Source: three-view drawing plus pictorial views. Frame: mm from the lowest corner of the part. Coordinates: 2 decimals unless noted, no trailing zeros. Write each loop counter-clockwise with the first axis right and the second up, starting at its lowest first coordinate (ties: lowest second). Pieces come first, ordered by that corner, then holes. Notation, with made-up numbers: (68.5, -20) - (99.5, -20) arc R19 ccw to (99.5, -1) - close; hole circle Ø3 at (-27, 53). An arc over 180 degrees is marked (long way). One line per item, written item: value.
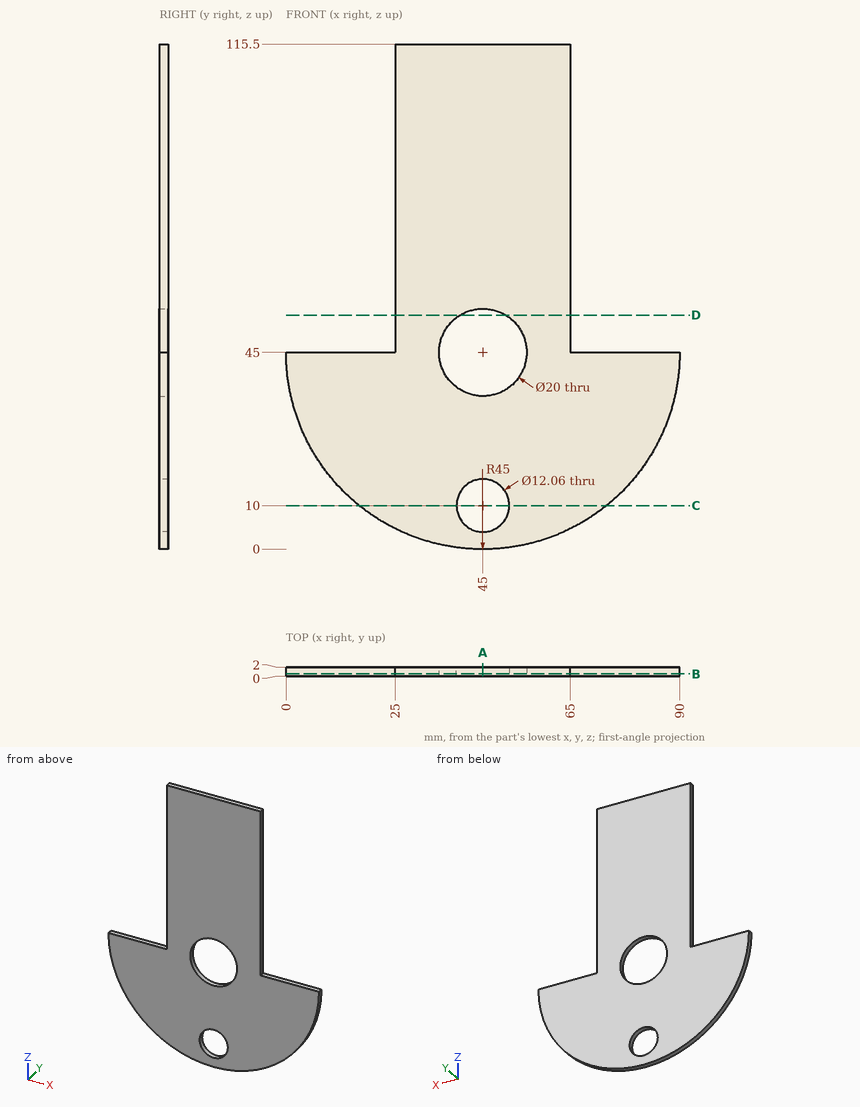
1) Material intervals for line 1 (Z direction, x = 45, y = 0.9); line 2 (X direction, y = 0.9, z = 53); line 3 (X direction, y = 0.85, z = 97), sorted ascending.
Values found:
line 1: 0 to 3.97, 16.03 to 35, 55 to 115.5
line 2: 25 to 39, 51 to 65
line 3: 25 to 65
2) Section query D-D on z = 53.5. Output: boundary loops of the cut face in (x, y), then the cut area to 3 significant figures.
Values found:
outline: (25, 0) - (39.73, 0) - (39.73, 2) - (25, 2) - close; (50.27, 0) - (65, 0) - (65, 2) - (50.27, 2) - close
area: 58.9 mm2
3) Section query B-B on y = 0.5. Output: boundary loops of the cut face in (x, z).
Values found:
outline: (0, 45) arc R45 ccw to (90, 45) - (65, 45) - (65, 115.5) - (25, 115.5) - (25, 45) - close; hole circle Ø20 at (45, 45); hole circle Ø12.06 at (45, 10)
4) Section query C-C on z = 10. Output: boundary loops of the cut face in (x, y), then the cut area to 3 significant figures.
Values found:
outline: (16.72, 0) - (38.97, 0) - (38.97, 2) - (16.72, 2) - close; (51.03, 0) - (73.28, 0) - (73.28, 2) - (51.03, 2) - close
area: 89.0 mm2
5) Section query A-A on x = 45. Output: boundary loops of the cut face in (y, z), then the cut area to 3 significant figures.
Values found:
outline: (0, 0) - (2, 0) - (2, 3.97) - (0, 3.97) - close; (0, 16.03) - (2, 16.03) - (2, 35) - (0, 35) - close; (0, 55) - (2, 55) - (2, 115.5) - (0, 115.5) - close
area: 167 mm2
